Part model, mm, in its own coordinate system. A direction names the side the tool comes from. Coordinates: 2 decimals unless noted, no trailing zeros. Write each loop counter-clockwise with the first axis right and the second up, starting at its lowest first coordinate (ties: lowest second). Pieces come first, ordered by that corner, then holes. Notation, with made-up numbers: (42, 82.25) -> (67, 82.25) arc R27 cw to (67, 115.25) -> close; hole circle Ø10 at (37.5, 68.5). An arc over 180 degrees is marked (long way). One line per question, with ' | ' between items. Start each with the question number.
Item 1: Probe probe 1 along X at (y, z) = (2, -0.25); probe 2 along Y at (x, z) = (-1, 3); probe 3 along Y at (x, z) = (-0.75, -5.75). List the from-to ranges inside material, lowest first. Write a range as [from, to].
Item 2: Saw through at C-C (x = 0). List the corners of the cut face in (y, z), and give its area (3 significant figures).
Item 3: Saw through at B-B (z = 2.75). List the corners of the cut face in (x, y).
Item 4: Pin check, flat tips, straight feed: pin 1 (2 mm diameter, centred on y = 19.5, z = 3.5, fed in from +X); pin 2 (5 mm diameter, centred on x = -1.5, y = 24.5, fed in from +Z); pin 3 (1.5 mm diameter, centred on x = -6, y = 6, fed in from +Z); pin 4 (4 mm diameter, centred on y = 20, z = -4, fed in from -X). Stop position of each tip, or through.
Item 5: Saw through at D-D (y = 9.5). List the corners of the cut face in (x, z), and give its area (3 significant figures).
Item 6: Saw through at A-A (y = -3.5). List the corners of the cut face in (x, z).
Item 7: 3-axis set-ups, long thin cutter, end or side, ignore diameter. For faces 1 (the flat face through (0, -2, 0)), 2 (the flat face through (0, 30, 0)), 3 (the cylindrical face through (-1.08, 14.79, -4.88)): which of +Z, -Z, +X, -X, +Y, -Y reach the whole face in a straight line?
from build123d import *

# Parameters (mm, degrees)
F0_R     = 5
F1_DEPTH = 30
F3_R     = 7.5
F4_DEPTH = 10
F7_DEPTH = 8


# Not quite as in the source:
# - a feature names something its author has since deleted; it is built from what else it names


with BuildPart() as f1:
    # F0 (on Front) → F1 (new body)
    with BuildSketch(Plane.XZ):
        Circle(F0_R)
    extrude(amount=-F1_DEPTH)

    # F3 (on offset) → F4 (join)
    with BuildSketch(Plane.XZ):
        Circle(F3_R)
    extrude(amount=F4_DEPTH)

    # F6 (on offset) → F7 (cut)
    with BuildSketch(Plane.XZ.offset(10)):
        Polygon((5, 0), (2.4813610619, 4.3408348599), (-2.5225813199, 4.3170109433), (-5, 0), (-2.5277935483, -4.313961031), (2.5273847237, -4.3142005584), align=None)
    extrude(amount=-F7_DEPTH, mode=Mode.SUBTRACT)


solid = f1.part
From the geometry:
1) probe 1: [-4.99, 4.99] | probe 2: [-2, 30] | probe 3: [-10, 0]
2) outline: (-10, -7.5) -> (0, -7.5) -> (0, -5) -> (30, -5) -> (30, 5) -> (0, 5) -> (0, 7.5) -> (-10, 7.5) -> (-10, 4.33) -> (-2, 4.33) -> (-2, -4.31) -> (-10, -4.31) -> close | area: 381 mm2
3) outline: (-6.98, -10) -> (-3.42, -10) -> (-3.42, -2) -> (3.4, -2) -> (3.4, -10) -> (6.98, -10) -> (6.98, 0) -> (4.18, 0) -> (4.18, 30) -> (-4.18, 30) -> (-4.18, 0) -> (-6.98, 0) -> close
4) pin 1: x = 4.33 | pin 2: z = 5 | pin 3: through | pin 4: x = -4.58
5) outline: circle Ø10 at (0, 0) | area: 78.5 mm2
6) outline: circle Ø15 at (0, 0); hole (-5, 0) -> (-2.53, -4.31) -> (2.53, -4.31) -> (5, 0) -> (2.48, 4.34) -> (-2.52, 4.32) -> close
7) face 1: -Y | face 2: +Z, -Z, +X, -X, +Y | face 3: +Y
